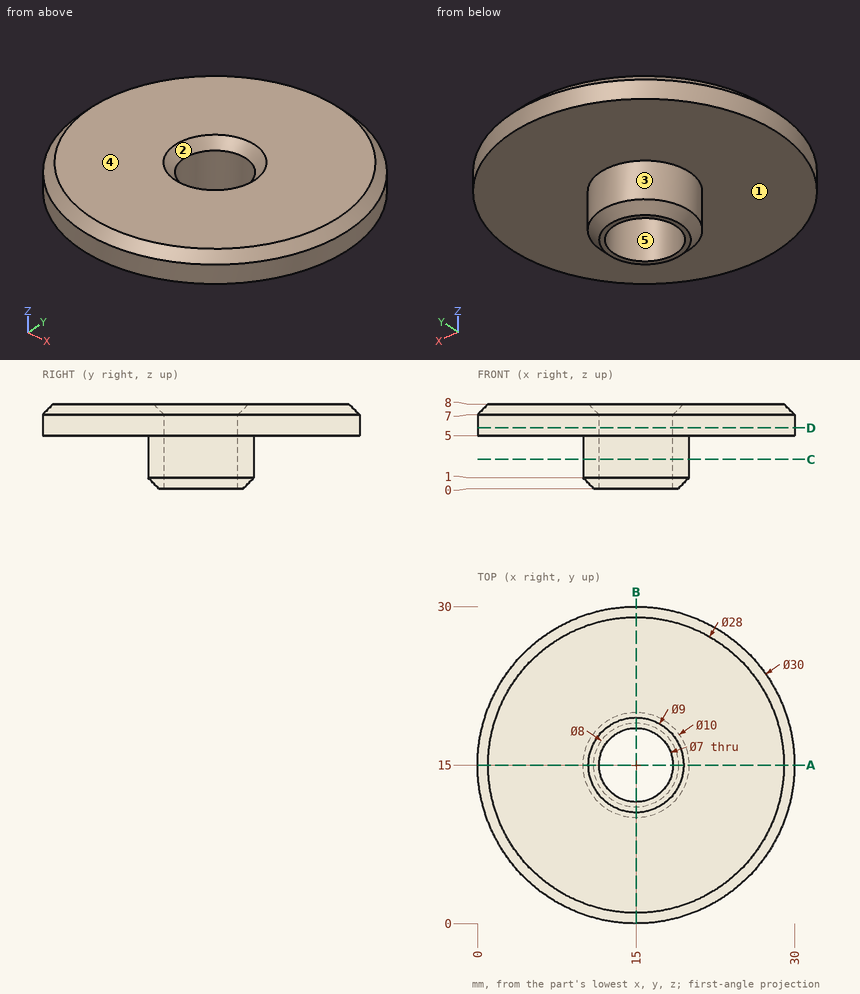
Verification items for this drawing (mm, ordinates from the low corner). A direction names the side the tool comes from. Coordinates: 2 decimals unless noted, no trailing zeros. Order: outer loops, then holes, each group sorted by start corner. A loop starts at its lowest first (then second) coordinate and runs counter-clockwise, first axis right, second up.
Q1. Tool access check on the marked faces 1 and 2. Record the directions out of +Z, -Z, +X, -X, +Y, -Y that give a thin tool (end or side, any length) a straight path to the whole face; none if there is none.
Reply:
face 1: -Z
face 2: +Z
Q2. Sectioned sample at D-D on z = 5.75. Record the cut outline in (x, y).
Reply:
outline: circle Ø30 at (15, 15); hole circle Ø7 at (15, 15)
Q3. Depth check by flat-ended pin: pin 1 Ø1.5 at (x, z) = (23.5, 3.5) entering from -Y; pin 2 Ø4 at (x, z) = (26, 7) entering from -Y; pin 3 Ø2 at (x, z) = (10.5, 6) entering from +Y. Enter the tip coordinate at first touch or a pass-through.
Reply:
pin 1: passes through
pin 2: stops at y = 3
pin 3: stops at y = 29.59
Q4. Draft check along X on the marked faces 3, 4 and 5. Enter one of: released by +X, released by -X, zero draft, split by the parting line, or undercut.
Reply:
face 3: split by the parting line
face 4: zero draft
face 5: undercut
Q5. Sectioned sample at C-C on z = 2.75. Record the cut outline in (x, y).
Reply:
outline: circle Ø10 at (15, 15); hole circle Ø7 at (15, 15)
Q6. Thickness scan on probe 1 along X at (y, z) = (15, 3); probe 2 along Y at (x, z) = (15, 5.5). Record the ranges inside material, lowest first.
Reply:
probe 1: x = 10 to 11.5, 18.5 to 20
probe 2: y = 0 to 11.5, 18.5 to 30
Q7. Sectioned sample at A-A on y = 15. Record the cut outline in (x, z).
Reply:
outline: (0, 5) - (10, 5) - (10, 1) - (11, 0) - (11.5, 0) - (11.5, 7) - (10.5, 8) - (1, 8) - (0, 7) - close; (18.5, 0) - (19, 0) - (20, 1) - (20, 5) - (30, 5) - (30, 7) - (29, 8) - (19.5, 8) - (18.5, 7) - close
